Work out the finished part from the listing and answer in its coordinate system (mm). Face numbers are marked on the shaded views. A direction names the side the tool comes from. Round coordinates to 2 decimals unless told otherwise and drop trailing zeros. Loops run counter-clockwise (first coordinate to the right, second up) from the corner with the lowest first, then second, coordinate; pieces in that order, holes last. Notation, with made-up numbers: (-11.5, 80.5) -> (20.5, 80.5) arc R21 ccw to (20.5, 113.5) -> close; hole circle Ø4 at (71.5, 60). An arc over 180 degrees is marked (long way). Write item = value, one per line. Start each with the question number.
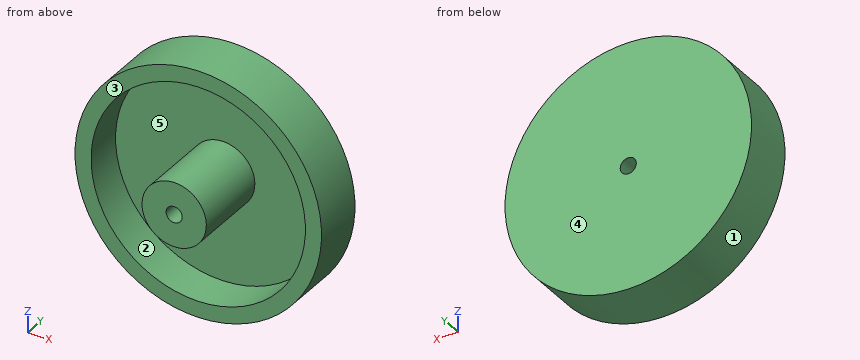
```python
from build123d import *

# Parameters (mm, degrees)
SKETCH1_R           = 23
BOSS_EXTRUDE1_DEPTH = 10
SKETCH2_R           = 20
CUT_EXTRUDE1_DEPTH  = 7.3
SKETCH3_R           = 6
BOSS_EXTRUDE3_DEPTH = 14.5
SKETCH4_R           = 1.5
CUT_EXTRUDE2_DEPTH  = 17.2


with BuildPart() as part:
    # Sketch1 → Boss-Extrude1 (new body)
    with BuildSketch(Plane(origin=(0, 0, 0), x_dir=(1, 0, 0), z_dir=(0, 1, 0))):
        with Locations(Location((0, 0, 0), (0, 0, 270))):
            Circle(SKETCH1_R)
    extrude(amount=BOSS_EXTRUDE1_DEPTH)

    # Sketch2 → Cut-Extrude1 (cut)
    with BuildSketch(Plane.XZ):
        with Locations(Location((0, 0, 0), (0, 0, 270))):
            Circle(SKETCH2_R)
    extrude(amount=-CUT_EXTRUDE1_DEPTH, mode=Mode.SUBTRACT)

    # Sketch3 → Boss-Extrude3 (add)
    with BuildSketch(Plane.XZ.offset(-7.3)):
        with Locations(Location((0, 0, 0), (0, 0, 90))):
            Circle(SKETCH3_R)
    extrude(amount=BOSS_EXTRUDE3_DEPTH)

    # Sketch4 → Cut-Extrude2 (cut)
    with BuildSketch(Plane.XZ.offset(7.2)):
        with Locations(Location((0, 0, 0), (0, 0, 270))):
            Circle(SKETCH4_R)
    extrude(amount=-CUT_EXTRUDE2_DEPTH, mode=Mode.SUBTRACT)


solid = part.part
```
Item 1: Find the intervals of material crossed by line 1 along X through (y, z) = (5, 0); line 2 along Z through (x, y) = (5, 4.5); line 3 along Y through (x, z) = (9, -18), in increasing order. Write a range as [from, to].
Item 2: Section C-C (x = -18.5) is taken. Determine the outline of the cut face in (y, z), then the cut area to 3 significant figures.
Item 3: Section D-D (z = -13) is taken. Determine the outline of the cut face in (x, y).
Item 4: The mould has two halves that part along Z. Classify the marked faces 1, 2 and 3: pulls with the +Z half, pulls with the -Z half, needs draft (parallel to the pull), parting line crosses it, or undercut.
Item 5: Flat-ended cylindrical pins translate along their axes: pin 1 (1.5 mm diameter, centred on x = -16, z = 12, fed in from -Y); pin 2 (6 mm diameter, centred on y = 8, z = 5.5, fed in from -X); pin 3 (10 mm diameter, centred on y = 3.5, z = -12.5, fed in from -X). Find the tip coordinate at first contact, or state that the pin passes through.
Item 6: Section B-B (z = 0) is taken. Determine the outline of the cut face in (x, y).
Item 7: Section A-A (x = 0) is taken. Determine the outline of the cut face in (y, z), then the cut area to 3 significant figures.
Item 8: A tool of negligible diameter and unlimited length cuts with its end or side. For the marked faces 4 and 5, from which of +Z, -Z, +X, -X, +Y, -Y can it reach the whole face along a straight path? Write none if from no direction.
Worked answers:
q1.line_1 = [-23, -20], [-6, -1.5], [1.5, 6], [20, 23]
q1.line_2 = [-22.45, -19.36], [-3.32, 3.32], [19.36, 22.45]
q1.line_3 = [0, 10]
q2.outline = (0, -13.67) -> (10, -13.67) -> (10, 13.67) -> (0, 13.67) -> (0, 7.6) -> (7.3, 7.6) -> (7.3, -7.6) -> (0, -7.6) -> close
q2.area = 162 mm2
q3.outline = (-18.97, 0) -> (-15.2, 0) -> (-15.2, 7.3) -> (15.2, 7.3) -> (15.2, 0) -> (18.97, 0) -> (18.97, 10) -> (-18.97, 10) -> close
q4.face_1 = parting line crosses it
q4.face_2 = undercut
q4.face_3 = needs draft
q5.pin_1 = 0
q5.pin_2 = -22.86
q5.pin_3 = -21.74
q6.outline = (-23, 0) -> (-20, 0) -> (-20, 7.3) -> (-6, 7.3) -> (-6, -7.2) -> (-1.5, -7.2) -> (-1.5, 10) -> (-23, 10) -> close; (1.5, -7.2) -> (6, -7.2) -> (6, 7.3) -> (20, 7.3) -> (20, 0) -> (23, 0) -> (23, 10) -> (1.5, 10) -> close
q7.outline = (-7.2, -6) -> (7.3, -6) -> (7.3, -20) -> (0, -20) -> (0, -23) -> (10, -23) -> (10, -1.5) -> (-7.2, -1.5) -> close; (-7.2, 1.5) -> (10, 1.5) -> (10, 23) -> (0, 23) -> (0, 20) -> (7.3, 20) -> (7.3, 6) -> (-7.2, 6) -> close
q7.area = 290 mm2
q8.face_4 = +Z, -Z, +X, -X, +Y
q8.face_5 = -Y
